```python
from build123d import *

# Parameters (mm, degrees)
F2_R          = 6
F3_DEPTH      = 25
F3_DEPTH_BACK = 25
F4_R          = 6
F5_DEPTH      = 25
F5_DEPTH_BACK = 25


with BuildPart() as f1:
    # F0 (on Front) → F1 (revolve)
    with BuildSketch(Plane.XZ):
        Polygon((14.75, 1.8402526621), (14.75, 0), (16, 0), (16, 1.8402526621), (12.959116371, 6.8669730598), (9.5678537413, 8.778959482), (0, 8.778959482), (0, 8.278959482), (8.0359548395, 8.278959482), (12.3140602287, 5.8669730598), align=None)
    revolve(axis=Axis((0, 0, 4.778959482), (0, 0, 1)))

    # F2 (on Front) → F3 (cut, two sides)
    with BuildSketch(Plane.XZ) as f3_sk:
        Circle(F2_R)
    extrude(amount=-F3_DEPTH, mode=Mode.SUBTRACT)
    extrude(f3_sk.sketch, amount=F3_DEPTH_BACK, mode=Mode.SUBTRACT)

    # F4 (on Right) → F5 (cut, two sides)
    with BuildSketch(Plane.YZ) as f5_sk:
        Circle(F4_R)
    extrude(amount=-F5_DEPTH, mode=Mode.SUBTRACT)
    extrude(f5_sk.sketch, amount=F5_DEPTH_BACK, mode=Mode.SUBTRACT)


solid = f1.part
```
For this review, take the finished solid that the model builds, in its own axes (mm). A direction names the side the tool comes from. Round coordinates to 2 decimals unless told otherwise and drop trailing zeros. Order: outer loops, then holes, each group sorted by start corner. A loop starts at its lowest first (then second) coordinate and runs counter-clockwise, first axis right, second up.
Q1. We need section B-B, the plane x = 0. Give the boundary of the cut face in (y, z).
Findings below:
outline: (-13.48, 6) - (-12.08, 6) - (-8.04, 8.28) - (8.04, 8.28) - (12.08, 6) - (13.48, 6) - (12.96, 6.87) - (9.57, 8.78) - (-9.57, 8.78) - (-12.96, 6.87) - close
Q2. We need section A-A, the plane z = 4.75. Give the boundary of the cut face in (x, y), plus the area to 3 significant figures.
Findings below:
outline: (-13.76, -3.67) arc R14.24 ccw to (-3.67, -13.76) - (-3.67, -12.46) arc R12.99 cw to (-12.46, -3.67) - close; (-13.76, 3.67) - (-12.46, 3.67) arc R12.99 cw to (-3.67, 12.46) - (-3.67, 13.76) arc R14.24 ccw to start; (3.67, -13.76) arc R14.24 ccw to (13.76, -3.67) - (12.46, -3.67) arc R12.99 cw to (3.67, -12.46) - close; (3.67, 12.46) arc R12.99 cw to (12.46, 3.67) - (13.76, 3.67) arc R14.24 ccw to (3.67, 13.76) - close
area: 69.8 mm2
Q3. Mouldability with a two-part tool opening along Y and no side actions: class faces 1 (the cylindrical face through (-10.37, 10.49, 0.91)), 2 (the cylindrical face through (-11.247, 11.38, 0.933)), 3 (the cylindrical face through (11.247, -11.38, 0.933)), 4 (the flat face through (11, -11, 0)) as pulls with the +Y half, pulls with the -Y half, needs draft (parallel to the pull), parting line crosses it, or undercut.
Findings below:
face 1: undercut
face 2: pulls with the +Y half
face 3: pulls with the -Y half
face 4: needs draft
Q4. Wall thickness on line 1 (Z direction, x = -1, y = 7); line 2 (X direction, y = -1.25, z = 6); line 3 (X direction, y = 5, z = 3.75): over which ranges is each line inside the solid? List them lowest first.
Findings below:
line 1: z = 8.28 to 8.78
line 2: x = -13.43 to -12.01, 12.01 to 13.43
line 3: x = -13.98 to -12.64, 12.64 to 13.98
Q5. Machinability: for faces 5 (the cylindrical face through (11.38, 11.247, 0.933)), 6 (the cylindrical face through (10.37, -10.49, 0.91)), which of the approach directions +Z, -Z, +X, -X, +Y, -Y give a long, thin tool a straight path to every point of the face, cutting with its end or side? Answer none if there is none.
Findings below:
face 5: +Z, -Z, +X, +Y
face 6: -Z
Q6. Insertion check: P1, Ø1, axis at x = 9.5, z = 1.5, coming from the +Y side; P2, Ø3, axis at y = -2, z = 6.5, coming from the -X side; P3, Ø5, axis at y = 2.5, z = 6.5, coming from the +X side. Each pin has a flat end and moves straight along its axis. Give the tip position at first contact, or say it passes through.
Findings below:
P1: stops at y = 13.23
P2: stops at x = -13.63
P3: stops at x = 13.84
Q7. We need section D-D, the plane z = 7.5. Give the boundary of the cut face in (x, y), plus the area to 3 significant figures.
Findings below:
outline: circle Ø23.67 at (0, 0); hole circle Ø18.84 at (0, 0)
area: 162 mm2
